For this review, take the finished solid that the model builds, in its own axes (mm). Face numbers are marked on the shaded views. A direction names the side the tool comes from. Give positions to 0.01 mm unless a question says otherwise; leave off trailing zeros. Write each loop counter-clockwise with the first axis right and the second up, starting at its lowest first coordinate (ties: lowest second). Pieces come first, ordered by that corner, then holes. Notation, with made-up numbers: M 33.25,20.25 L 40.25,20.25 A8 ccw 40.25,25.25 Z; hole C 42.25,56.5 d6. An arc over 180 degrees is marked long. Write item = value, one per line.
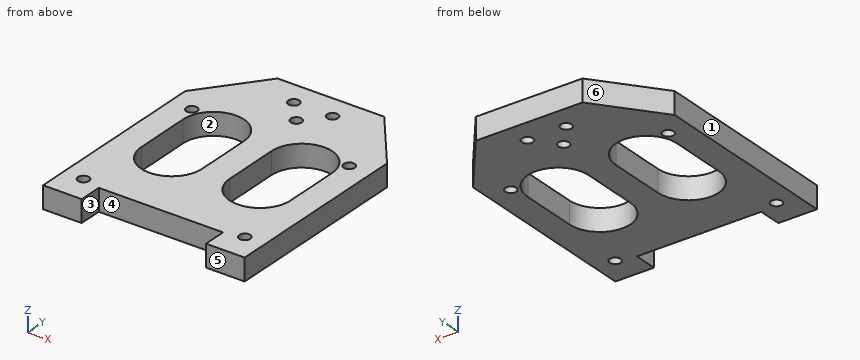
```python
from build123d import *

# Parameters (mm, degrees)
ESBO_O2_R                = 2
RESSALTO_EXTRUS_O1_DEPTH = 8


with BuildPart() as part:
    # Esboço2 → Ressalto-extrusão1 (new body)
    with BuildSketch(Plane.XY):
        Polygon((36.5, -75), (36.5, -5), (19.311716217, 17), (-19.311716217, 17), (-36.5, -5), (-36.5, -75), (-22.499999998, -75), (-22.499999998, -66.599999996), (22.499999998, -66.599999996), (22.499999998, -75), align=None)
        with Locations((28.5, -12.7)):
            Circle(ESBO_O2_R, mode=Mode.SUBTRACT)
        with Locations((29.2, -65)):
            Circle(ESBO_O2_R, mode=Mode.SUBTRACT)
        with Locations((-29.2, -65)):
            Circle(ESBO_O2_R, mode=Mode.SUBTRACT)
        with Locations((-28.5, -12.7)):
            Circle(ESBO_O2_R, mode=Mode.SUBTRACT)
        with Locations((7, 8.3)):
            Circle(ESBO_O2_R, mode=Mode.SUBTRACT)
        with Locations((-7, 8.3)):
            Circle(ESBO_O2_R, mode=Mode.SUBTRACT)
        Circle(ESBO_O2_R, mode=Mode.SUBTRACT)
        with BuildLine():
            ThreePointArc((5.030193795, -39.591075239), (16.030188189, -50.591069634), (27.030182584, -39.591075239))
            Line((27.030182584, -39.591075239), (27.030169807, -19.087507994))
            ThreePointArc((27.030169807, -19.087507994), (16.030168558, -8.087513599), (5.030181018, -19.087507994))
            Line((5.030181018, -19.087507994), (5.030193795, -39.591075239))
        make_face(mode=Mode.SUBTRACT)
        with BuildLine():
            ThreePointArc((-26.977366802, -39.591075239), (-15.977372644, -50.591069397), (-4.977378486, -39.591075239))
            Line((-4.977378486, -39.591075239), (-4.977391172, -19.009684113))
            ThreePointArc((-4.977391172, -19.009684113), (-15.977385329, -8.009689955), (-26.977379487, -19.009684113))
            Line((-26.977379487, -19.009684113), (-26.977366802, -39.591075239))
        make_face(mode=Mode.SUBTRACT)
    extrude(amount=RESSALTO_EXTRUS_O1_DEPTH)


solid = part.part
```
1. We need section D-D, the plane x = -28.5. Write out the cut boundary in (y, z), then the cut area to 3 significant figures.
Responses:
outline = M -75,0 L -66.87,0 L -66.87,8 L -75,8 Z; M -63.13,0 L -14.7,0 L -14.7,8 L -63.13,8 Z; M -10.7,0 L 5.24,0 L 5.24,8 L -10.7,8 Z
area = 580 mm2
2. Machinability: for the marked faces 1, 2 and 3, which of the approach directions +Z, -Z, +X, -X, +Y, -Y give a long, thin tool a straight path to every point of the face, cutting with its end or side? Answer none if there is none.
Responses:
face_1 = +Z, -Z, -X, +Y, -Y
face_2 = +Z, -Z
face_3 = +Z, -Z, -Y
3. The part is to be moulded in two halves that separate along X. For the marked faces 4, 5 and 6, say which applies: +X half, -X half, draft (parallel to the pull), parting line (faces both ways), or undercut.
Responses:
face_4 = undercut
face_5 = draft
face_6 = -X half
4. We need section C-C, the plane z = 3.5. Count the separate pieces of the cut face and the enclosed holes in it, then the cut area to 3 significant figures.
Responses:
separate_pieces = 1
enclosed_holes = 9
area = 4,210 mm2
5. Insertion check: P1, Ø3.5, axis at x = -29.2, y = -65, coming from the +Z side; P2, Ø6.5, axis at x = 0, y = 0, coming from the -Z side; P3, Ø3, axis at x = 10, z = 3.5, coming from the -Y side. Each pin has a flat end and moves straight along its axis. Give the tip position at first contact, or say it passes through.
Responses:
P1 = through
P2 = 0
P3 = -66.6
6. We need section A-A, the plane x = 0. Write out the cut boundary in (y, z).
Responses:
outline = M -66.6,0 L -2,0 L -2,8 L -66.6,8 Z; M 2,0 L 17,0 L 17,8 L 2,8 Z
7. For line 1 along X through (y, z) = (-34, 3.75); line 2 along Y through (x, z) = (-6.5, 1); line 3 along Y through (x, z) = (0, 4.5), list the stretches that pass through material, from the lowest coordinate up. Write a range as from..to.
Responses:
line_1 = -36.5..-26.98, -4.98..5.03, 27.03..36.5
line_2 = -66.6..-45.17, -13.43..6.36, 10.24..17
line_3 = -66.6..-2, 2..17
8. We need section B-B, the plane y = -21. Write out the cut boundary in (x, z), then the cut area to 3 significant figures.
Responses:
outline = M -36.5,0 L -26.98,0 L -26.98,8 L -36.5,8 Z; M -4.98,0 L 5.03,0 L 5.03,8 L -4.98,8 Z; M 27.03,0 L 36.5,0 L 36.5,8 L 27.03,8 Z
area = 232 mm2
